Source: CAD feature listing. Evaluate the final solid. Frame: model axes, mm. Face numbers are marked on the shaded views. A direction names the side the tool comes from. Give positions to 0.01 mm unless a question says otherwise; leave off trailing zeros. Order: outer loops, then holes, each group sorted by start corner. A loop starts at its lowest first (then second) coordinate and runs counter-clockwise, first axis right, second up. Notation, with made-up numbers: M 60.25,-39.75 L 66.25,-39.75 A11 ccw 66.25,-26.75 Z; hole C 87,-15 d6. An arc over 180 degrees is marked long. Answer in a Markdown table with one row per item. Add a question column.
(1) Section query C-C, the plane x = -4. Return loops of the section in (y, z).
(2) Material intervals for line 1 along Z through (x, y) = (-34, 0); line 2 along Y through (x, z) = (-17, 0); line 3 along Z through (x, y) = (-10, 0), sorted ascending.
(3) Section query D-D, the plane z = -21.5. Return loops of the section in (x, y).
(4) Pin query (flat end, axial travel): P1, Ø4, axis at x = -41, z = -18, coming from the +Y side; P2, Ø2, axis at y = 5.5, z = 12, coming from the +X side; P3, Ø4, axis at x = -36, y = 31.5, coming from the -Z side; P4, Ø18, axis at y = 0, z = 0, coming from the +X side. Return the tip coordinate at first contact, or that it passes through.
(5) Mould query, pull axis Y, two halves, no side actions, for the marked faces 4, 5 and 6. Classes: pulls with the +Y half, pulls with the -Y half, needs draft (parallel to the pull), parting line crosses it, or undercut.
(6) Set-up query: the marked faces 1, 2 and 3. Return all of +Z, -Z, +X, -X, +Y, -Y with unobstructed straight access to the full face (end or side cutting, diameter ignored); none if empty.
from build123d import *

# Parameters (mm, degrees)
F0_W    = 40
F0_H    = 15
F2_SIZE = 0.99999


# Not quite as in the source:
# - a fillet or chamfer is up to 0.001 mm smaller than in the source, because OpenCascade refuses the exact size


with BuildPart() as f1:
    # F0 (on Front) → F1 (revolve)
    with BuildSketch(Plane.XZ):
        Polygon((-45, 40), (-50, 40), (-50, 14), (-40, 14), (-40, 12.5), (-25, 12.5), (-25, 14), (-15, 14), (-15, 15), (0, 15), (0, 40), (-5, 40), (-5, 25), (-45, 25), align=None)
        with Locations((-25, 32.5)):
            Rectangle(F0_W, F0_H)
    revolve(axis=Axis((-17.5871104002, 0, 0), (1, 0, 0)))

    # F2 (size 1 in the source; OpenCascade refuses exactly that, so slightly less here)
    f2_edges = [f1.edges().sort_by_distance(p)[0] for p in [
        (-15, 0, -14),
        (-50, 0, -14),
    ]]
    chamfer(f2_edges, length=F2_SIZE)


solid = f1.part
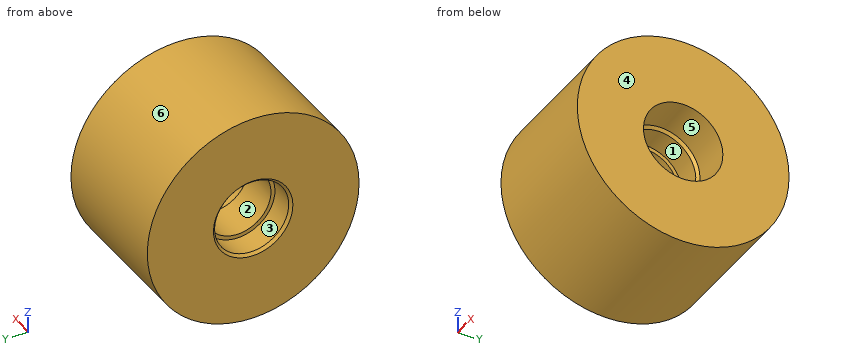
Values follow:
| question | item | result |
|---|---|---|
| 1 | outline | C 0,0 d80; hole C 0,0 d30 |
| 2 | line 1 | z = -40 to -12.5, 12.5 to 40 |
| 2 | line 2 | y = -40 to -14, 14 to 40 |
| 2 | line 3 | z = -40 to -15, 15 to 40 |
| 3 | outline | M -50,-33.73 L 0,-33.73 L 0,33.73 L -50,33.73 Z |
| 4 | P1 | stops at y = 36.66 |
| 4 | P2 | stops at x = -15.8 |
| 4 | P3 | stops at z = -27.01 |
| 4 | P4 | passes through |
| 5 | face 4 | needs draft |
| 5 | face 5 | undercut |
| 5 | face 6 | parting line crosses it |
| 6 | face 1 | +X |
| 6 | face 2 | +X, -X |
| 6 | face 3 | -X |
